Geometry check sheet. Reference: the model listing, model coordinates, mm. Coordinates: 2 decimals unless noted, no trailing zeros. Order: outer loops, then holes, each group sorted by start corner. A loop starts at its lowest first (then second) coordinate and runs counter-clockwise, first axis right, second up. Notation, with made-up numbers: M -36.5,-31 L 17.5,-31 A14 cw 17.5,-26 Z; hole C 1,-13.5 d11. An arc over 180 degrees is marked long. One line per item, written item: value. Start each with the question number.
1) Sectioned sample at D-D, the plane z = -3.25. Enter the section's corners in (x, y), then the cut area to 3 significant figures.
2) Sectioned sample at A-A, the plane x = -12.5. Enter the section's corners in (y, z), then the cut area to 3 significant figures.
3) Go/stop test with a flat-tipped pin: P1, Ø5, axis at x = 22.5, z = -0.5, coming from the -Y side. Record where the tip stops, or that it passes through.
4) Sectioned sample at C-C, the plane z = 0. Enter the section's corners in (x, y).
5) Sectioned sample at B-B, the plane y = -1.3. Enter the section's corners in (x, z).
6) Thickness scan on L1, parallel to Y at x = -34, z = 1; L2, parallel to Z at x = 12, y = -2.2; L3, parallel to Z at x = -7.5, y = -2.4. Record the ranges inside material, lowest first. Write a range as from..to.
7) Draft check along Z on faces 1 (the flat face through (43, -0.27, -0.03)), 2 (the cylindrical face through (0.602, -0.886, -6.923)), 3 (the cylindrical face through (0.6, -0.43, -0.08)), 4 (the cylindrical face through (1, 0, 0)). Enter one of: pulls with the +Z half, pulls with the -Z half, needs draft (parallel to the pull), parting line crosses it, or undercut.
```python
from build123d import *

# Parameters (mm, degrees)
BOSS_EXTRUDE1_DEPTH = 43


with BuildPart() as part:
    # Sketch1 → Boss-Extrude1 (new body, symmetric)
    with BuildSketch(Plane(origin=(0, 0, 0), x_dir=(0, 0, -1), z_dir=(1, 0, 0))):
        with BuildLine():
            Line((6.678248915, -2.066776115), (5.793546079, -2.951478951))
            Line((5.793546079, -2.951478951), (5.489490163, -2.647423035))
            Line((5.489490163, -2.647423035), (6.374192999, -1.762720199))
            ThreePointArc((6.374192999, -1.762720199), (6.527082765, -1.0543294), (5.944808192, -0.622879372))
            ThreePointArc((5.944808192, -0.622879372), (0, -0.43), (-5.944808192, -0.622879372))
            ThreePointArc((-5.944808192, -0.622879372), (-6.527082765, -1.0543294), (-6.374192999, -1.762720199))
            Line((-6.374192999, -1.762720199), (-5.489490163, -2.647423035))
            Line((-5.489490163, -2.647423035), (-5.793546079, -2.951478951))
            Line((-5.793546079, -2.951478951), (-6.678248915, -2.066776115))
            ThreePointArc((-6.678248915, -2.066776115), (-6.929478176, -0.902744659), (-5.97268156, -0.193783724))
            ThreePointArc((-5.97268156, -0.193783724), (0, 0), (5.97268156, -0.193783724))
            ThreePointArc((5.97268156, -0.193783724), (6.929478176, -0.902744659), (6.678248915, -2.066776115))
        make_face()
    extrude(amount=BOSS_EXTRUDE1_DEPTH, both=True)


solid = part.part
```
Final values:
1. outline: M -43,-0.49 L 43,-0.49 L 43,-0.06 L -43,-0.06 Z
1. area: 37.0 mm^2
2. outline: M -2.95,-5.79 L -2.07,-6.68 A1.1 ccw -0.19,-5.97 A92.14 ccw -0.19,5.97 A1.1 ccw -2.07,6.68 L -2.95,5.79 L -2.65,5.49 L -1.76,6.37 A0.67 cw -0.62,5.94 A91.71 cw -0.62,-5.94 A0.67 cw -1.76,-6.37 L -2.65,-5.49 Z
2. area: 7.95 mm^2
3. P1: stops at y = -0.48
4. outline: M -43,-0.43 L 43,-0.43 L 43,0 L -43,0 Z
5. outline: M -43,-7 L 43,-7 L 43,-6.57 L -43,-6.57 Z; M -43,6.57 L 43,6.57 L 43,7 L -43,7 Z
6. L1: y = -0.44..-0.01
6. L2: z = -6.55..-5.94, 5.94..6.55
6. L3: z = -6.35..-5.74, 5.74..6.35
7. face 1: needs draft
7. face 2: pulls with the -Z half
7. face 3: undercut
7. face 4: parting line crosses it
